Could you check a few things on this drawing? It's one solid part, dimensions in mm from its lowest x, y, z. A direction names the side the tool comes from. Coordinates: 2 decimals unless noted, no trailing zeros. Write each loop counter-clockwise with the first axis right and the second up, starting at its lowest first coordinate (ties: lowest second). Pieces come first, ordered by that corner, then holes.
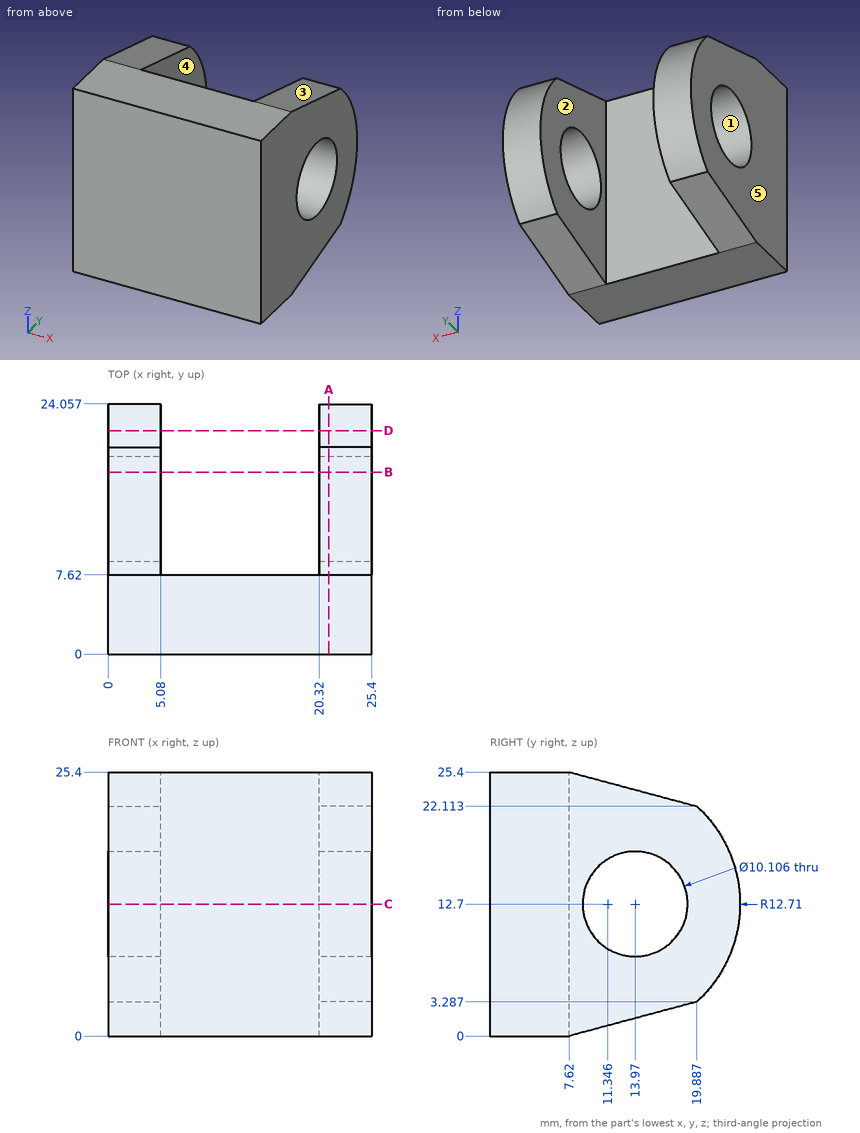
1) Imagine slicing it at D-D on y = 21.5. Please give me the cut outline in (x, z) (1 decimal).
Values follow:
outline: (0, 5.1) - (5.1, 5.1) - (5.1, 20.3) - (0, 20.3) - close; (20.3, 5.1) - (25.4, 5.1) - (25.4, 20.3) - (20.3, 20.3) - close
2) On a 3-axis mill with a long thin cutter (end or side, diameter ignored), from which of +Z, -Z, +X, -X, +Y, -Y can I reach the whole of each face in a straight line? I mean the marked faces 4 and 5. Say none if no direction works.
Values follow:
face 4: +Z, -Z, +Y
face 5: +Z, -Z, -X, +Y, -Y
3) Imagine slicing it at C-C on z = 12.7. Please give me the cut outline in (x, y).
Values follow:
outline: (0, 0) - (25.4, 0) - (25.4, 8.92) - (20.32, 8.92) - (20.32, 7.62) - (5.08, 7.62) - (5.08, 8.92) - (0, 8.92) - close; (0, 19.02) - (5.08, 19.02) - (5.08, 24.06) - (0, 24.06) - close; (20.32, 19.02) - (25.4, 19.02) - (25.4, 24.06) - (20.32, 24.06) - close
4) I need wall thicknesses on probe 1 along X at (y, z) = (20.25, 12.25); probe 2 along Y at (x, z) = (1.3, 12.7); probe 3 along Y at (x, z) = (21.25, 14.5). Which ranges of each line are inside material? Lowest first, please.
Values follow:
probe 1: x = 0 to 5.08, 20.32 to 25.4
probe 2: y = 0 to 8.92, 19.02 to 24.06
probe 3: y = 0 to 9.25, 18.69 to 23.93
5) Will these pins go through, and if not, where does the flat tip stop? pin 1 (3 mm diameter, centred on x = 13, z = 11.5, fed in from +Y); pin 2 (1.5 mm diameter, centred on x = 23, y = 11, fed in from -Z) (1 decimal); pin 3 (9 mm diameter, centred on y = 13.97, z = 12.7, fed in from +X); pin 4 (8 mm diameter, centred on x = 22, y = 15.5, fed in from -Z).
Values follow:
pin 1: stops at y = 7.62
pin 2: stops at z = 0.7
pin 3: passes through
pin 4: stops at z = 1.04
6) We'd pull the mould along Z, two halves only. Please class the marked faces 1, 2 and 3: pulls with the +Z half, pulls with the -Z half, needs draft (parallel to the pull), parting line crosses it, or undercut.
Values follow:
face 1: undercut
face 2: needs draft
face 3: pulls with the +Z half
7) Imagine slicing it at B-B on y = 17.5. Please give me the cut outline in (x, z) (1 decimal), then the cut area to 3 significant figures.
Values follow:
outline: (0, 2.6) - (5.1, 2.6) - (5.1, 9.1) - (0, 9.1) - close; (0, 16.3) - (5.1, 16.3) - (5.1, 22.8) - (0, 22.8) - close; (20.3, 2.6) - (25.4, 2.6) - (25.4, 9.1) - (20.3, 9.1) - close; (20.3, 16.3) - (25.4, 16.3) - (25.4, 22.8) - (20.3, 22.8) - close
area: 131 mm2
8) Imagine slicing it at A-A on x = 21.25. Please give me the cut outline in (y, z), then the cut area to 3 significant figures.
Values follow:
outline: (0, 0) - (7.62, 0) - (19.89, 3.29) arc R12.71 ccw to (19.89, 22.11) - (7.62, 25.4) - (0, 25.4) - close; hole circle Ø10.11 at (13.97, 12.7)
area: 439 mm2
